from build123d import *

# Parameters (mm, degrees)
F1_DEPTH = 3
F2_R     = 1


# Not quite as in the source:
# - a feature names something its author has since deleted; it is built from what else it names


with BuildPart() as f1:
    # F0 (on Top) → F1 (new body, symmetric)
    with BuildSketch(Plane.XY):
        with BuildLine():
            Line((-12.9470113486, 10.248668018), (-11.7864680784, 8.248668018))
            ThreePointArc((-11.7864680784, 8.248668018), (-7.2595115052, 2.3329471863), (-8.5698451786, -5))
            Line((-8.5698451786, -5), (8.5698451786, -5))
            ThreePointArc((8.5698451786, -5), (7.2595115052, 2.3329471863), (11.7864680784, 8.248668018))
            Line((11.7864680784, 8.248668018), (12.9470113486, 10.248668018))
            Line((12.9470113486, 10.248668018), (10.9470113486, 10.248668018))
            ThreePointArc((10.9470113486, 10.248668018), (0, 7.2662124228), (-10.9470113486, 10.248668018))
            Line((-10.9470113486, 10.248668018), (-12.9470113486, 10.248668018))
        make_face()
    extrude(amount=F1_DEPTH, both=True)

    # F2
    f2_edges = [f1.edges().sort_by_distance(p)[0] for p in [
        (-12.947011, 10.248668, 0),
        (12.947011, 10.248668, 0),
        (-8.569845, -5, 0),
        (8.569845, -5, 0),
    ]]
    fillet(f2_edges, radius=F2_R)


solid = f1.part
Can you work these out from the model? Positions are in its coordinate system, mm. Round coordinates to 2 decimals unless told otherwise and drop trailing zeros. Order: outer loops, then holes, each group sorted by start corner. A loop starts at its lowest first (then second) coordinate and runs counter-clockwise, first axis right, second up. Notation, with made-up numbers: (53, 38) - (78, 38) arc R16 ccw to (78, 55) - close; hole circle Ø1 at (25, -15.75). An arc over 180 degrees is marked (long way). Answer in a Markdown table with one row per item.
(1) Suppose I cut it at A-A, the plane x = -7.5. Please give me the cut outline in (y, z).
From the geometry:
| item | result |
|---|---|
| outline | (-4.78, -3) - (-2.85, -3) - (-2.85, 3) - (-4.78, 3) - close; (3.16, -3) - (8.61, -3) - (8.61, 3) - (3.16, 3) - close |
(2) For P1, Ø1, axis at x = -8.5, z = 1.5, coming from the -Y side; P2, Ø1, axis at y = -1.5, z = 2, coming from the +X side, each with a flat end and sliding along its axis, tell me the tip position at first contact or that it passes through.
From the geometry:
| item | result |
|---|---|
| P1 | stops at y = 4.34 |
| P2 | stops at x = 7.25 |
(3) Suppose I cut it at D-D, the plane y = -4. Please give me the cut outline in (x, z).
From the geometry:
| item | result |
|---|---|
| outline | (-7.88, -3) - (7.88, -3) - (7.88, 3) - (-7.88, 3) - close |
(4) Please list where these lines run through material, in increasing order: L1, parallel to X at y = 0.25, z = 2.75; L2, parallel to X at y = 9.75, z = 1.15; L3, parallel to Y at x = -8.75, z = -0.6. Write a range as from..to.
From the geometry:
| item | result |
|---|---|
| L1 | x = -7..7 |
| L2 | x = -12.08..-10.05, 10.05..12.08 |
| L3 | y = 5.57..9.12 |
(5) If we mould it in two halves opening along Y, with no side actions, what happens to faces 1 (the face through (12.07, 9.76, 0.04)), 2 (the face through (0.161, 7.267, 0.042)), 3 (the face through (-7.71, -4.56, 0.04)), 4 (the face through (0, 3, 3))? For each: released by +Y, released by -Y, zero draft, split by the parting line, or undercut.
From the geometry:
| item | result |
|---|---|
| face 1 | split by the parting line |
| face 2 | released by +Y |
| face 3 | undercut |
| face 4 | zero draft |
(6) Suppose I cut it at B-B, the plane z = 1.65. Please give me the cut outline in (x, y).
From the geometry:
| item | result |
|---|---|
| outline | (-12.08, 8.75) - (-11.79, 8.25) arc R9.24 cw to (-7.79, -3.59) arc R1 ccw to (-6.88, -5) - (6.88, -5) arc R1 ccw to (7.79, -3.59) arc R9.24 cw to (11.79, 8.25) - (12.08, 8.75) arc R1 ccw to (11.21, 10.25) - (10.95, 10.25) arc R21.58 cw to (-10.95, 10.25) - (-11.21, 10.25) arc R1 ccw to start |
(7) Suppose I cut it at C-C, the plane y = 7.75. Please give me the cut outline in (x, z).
From the geometry:
| item | result |
|---|---|
| outline | (-10.98, -3) - (-4.54, -3) - (-4.54, 3) - (-10.98, 3) - close; (4.54, -3) - (10.98, -3) - (10.98, 3) - (4.54, 3) - close |
